from build123d import *

# Parameters (mm, degrees)
SKETCH1_R           = 6
BOSS_EXTRUDE1_DEPTH = 19
SKETCH2_R           = 6
CUT_EXTRUDE1_DEPTH  = 12


with BuildPart() as part:
    # Sketch1 → Boss-Extrude1 (new, symmetric)
    with BuildSketch(Plane(origin=(0, 0, 0), x_dir=(1, 0, 0), z_dir=(0, 1, 0))):
        with BuildLine():
            Line((-25, 12.5), (25, 12.5))
            ThreePointArc((25, 12.5), (37.5, 0), (25, -12.5))
            Line((25, -12.5), (-25, -12.5))
            ThreePointArc((-25, -12.5), (-37.5, 0), (-25, 12.5))
        make_face()
        with Locations(Location((-25, 0, 0), (0, 0, 270))):
            Circle(SKETCH1_R, mode=Mode.SUBTRACT)
        with Locations(Location((25, 0, 0), (0, 0, 270))):
            Circle(SKETCH1_R, mode=Mode.SUBTRACT)
    extrude(amount=BOSS_EXTRUDE1_DEPTH, both=True)

    # Sketch2 → Cut-Extrude1 (cut)
    with BuildSketch(Plane.XY.offset(12.5)):
        Circle(SKETCH2_R)
    extrude(amount=-CUT_EXTRUDE1_DEPTH, mode=Mode.SUBTRACT)


solid = part.part
Source: CAD feature listing. Evaluate the final solid. Frame: model axes, mm. A direction names the side the tool comes from. Round coordinates to 2 decimals unless told otherwise and drop trailing zeros. Loops run counter-clockwise (first coordinate to the right, second up) from the corner with the lowest first, then second, coordinate; pieces in that order, holes last. Notation, with made-up numbers: (-32.75, 74) - (-7.75, 74) arc R22 ccw to (-7.75, 105) - close; hole circle Ø4 at (27, -33.75). An arc over 180 degrees is marked (long way). Write item = value, one per line. Start each with the question number.
Item 1: Section query C-C on x = 0. Output: boundary loops of the cut face in (y, z), plus the area to 3 significant figures.
Item 2: First-contact query: pin 1 Ø3 at (x, y) = (-28, -11) entering from -Z; pin 2 Ø2 at (y, z) = (9.5, -5) entering from -X; pin 3 Ø9.5 at (x, z) = (25, 0) entering from +Y; pin 4 Ø12 at (y, z) = (-14.5, 8.5) entering from +X. Flat tips, straight axial feed; report the tip coordinate or a pass-through.
Item 3: Section query D-D on y = 0. Output: boundary loops of the cut face in (x, z).
Item 4: Section query B-B on z = -0.75. Output: boundary loops of the cut face in (x, y), plus the area to 3 significant figures.
Item 5: Section query A-A on y = 12. Output: boundary loops of the cut face in (x, z).
Item 6: Material intervals for line 1 (X direction, y = -2.5, z = 0); line 2 (Y direction, x = 0, z = 5.5); line 3 (X direction, y = 8, z = -2.5), sorted ascending.
Item 7: Reachability of faces 4 (the face through (-6, 0, 7)), 5 (the face through (19.677, -0.266, 2.769)) from +Z, -Z, +X, -X, +Y, -Y: full face, straight path, thin tool, end or side. Return the list, or none.
Item 8: Mould query, pull axis X, two halves, no side actions, for faces 1 (the face through (-30.323, -0.266, 2.769)), 2 (the face through (1, -19, 0)), 3 (the face through (37.497, 0.266, -0.275)). Classes: released by +X, released by -X, zero draft, split by the parting line, or undercut.
Results list:
q1.outline = (-19, -12.5) - (19, -12.5) - (19, 12.5) - (6, 12.5) - (6, 0.5) - (-6, 0.5) - (-6, 12.5) - (-19, 12.5) - close
q1.area = 806 mm²
q2.pin_1 = -12.41
q2.pin_2 = -36.84
q2.pin_3 = through
q2.pin_4 = 37.25
q3.outline = (-25, -12.5) - (25, -12.5) arc R12.5 ccw to (25, 12.5) - (6, 12.5) - (6, 0.5) - (-6, 0.5) - (-6, 12.5) - (-25, 12.5) arc R12.5 ccw to start; hole circle Ø12 at (-25, 0); hole circle Ø12 at (25, 0)
q4.outline = (-37.48, -19) - (-30.95, -19) - (-30.95, 19) - (-37.48, 19) - close; (-19.05, -19) - (19.05, -19) - (19.05, 19) - (-19.05, 19) - close; (30.95, -19) - (37.48, -19) - (37.48, 19) - (30.95, 19) - close
q4.area = 1,940 mm²
q5.outline = (-25, -12.5) - (25, -12.5) arc R12.5 ccw to (25, 12.5) - (-25, 12.5) arc R12.5 ccw to start; hole circle Ø12 at (-25, 0); hole circle Ø12 at (25, 0)
q6.line_1 = -37.5 to -31, -19 to 19, 31 to 37.5
q6.line_2 = -19 to -6, 6 to 19
q6.line_3 = -37.25 to -30.45, -19.55 to 19.55, 30.45 to 37.25
q7.face_4 = +Z
q7.face_5 = +Y, -Y
q8.face_1 = undercut
q8.face_2 = zero draft
q8.face_3 = released by +X
